Autodesk Inventor part; units mm, degrees
ref_plane "YZ Plane" through (0, 0, 0) normal (1, 0, 0) x (0, 1, 0)
ref_plane "XZ Plane" through (0, 0, 0) normal (0, 1, 0) x (-1, 0, 0)
ref_plane "XY Plane" through (0, 0, 0) normal (0, 0, 1) x (1, 0, 0)
sketch "Sketch1" plane through (0, 0, 0) normal (0, 0, 1) x (1, 0, 0)
  line L0 (-16, 16) -> (16, 16)
  line L1 (16, 16) -> (16, -16)
  line L2 (16, -16) -> (-16, -16)
  line L3 (-16, -16) -> (-16, 16)
  point P0 (0, 0)
  dimension "d0" = 32
  dimension "d1" = 32
  dimension "d2" = 16
  dimension "d3" = 16
extrude "Firkant" add sketch "Sketch1" along normal blind 6
sketch "Sketch2" plane through (0, 0, 6) normal (0, 0, 1) x (1, 0, 0)
  circle A0 centre (0, 0) radius 10.5
  dimension "d6" = 21
extrude "Rør" add sketch "Sketch2" along normal blind 51
sketch "Sketch3" plane through (0, 0, 0) normal (0, 0, -1) x (-1, 0, 0)
  circle A0 centre (0, 0) radius 6
  dimension "d9" = 12
extrude "Hul" cut sketch "Sketch3" against normal up to surface (57 mm away)
sketch "Sketch4" plane through (0, 0, 6) normal (0, 0, 1) x (1, 0, 0)
  circle A0 centre (0, 0) radius 10.5 construction
  circle A1 centre (0, 0) radius 16 construction
  line L0 (-16, 16) -> (16, -16) construction
  line L1 (16, 16) -> (-16, -16) construction
  circle A2 centre (11.3137, 11.3137) radius 2.25
  circle A3 centre (-11.3137, 11.3137) radius 2.25
  circle A4 centre (-11.3137, -11.3137) radius 2.25
  circle A5 centre (11.3137, -11.3137) radius 2.25
  dimension "d12" = 32
  dimension "d13" = 4.5
  dimension "d14" = 4.5
  dimension "d15" = 4.5
  dimension "d16" = 4.5
extrude "d1 Hullerne (små)" cut sketch "Sketch4" against normal up to surface (6 mm away)
sketch "Sketch5" plane through (0, 0, 0) normal (0, 0, -1) x (-1, 0, 0)
  circle A0 centre (11.3137, -11.3137) radius 2.25
  circle A1 centre (-11.3137, -11.3137) radius 2.25
  circle A2 centre (11.3137, 11.3137) radius 2.25
  circle A3 centre (-11.3137, 11.3137) radius 2.25
  circle A4 centre (-11.3137, 11.3137) radius 4
  circle A5 centre (11.3137, 11.3137) radius 4
  circle A6 centre (11.3137, -11.3137) radius 4
  circle A7 centre (-11.3137, -11.3137) radius 4
  dimension "d19" = 8
  dimension "d20" = 8
  dimension "d21" = 8
  dimension "d22" = 8
extrude "d2 Hullerne (store)" cut sketch "Sketch5" against normal blind 4.4
chamfer "Hjørnerne" distance 3 angle 45 4 edges at (-16, -16, 3) (16, -16, 3) (16, 16, 3) (-16, 16, 3)
equation "\"d1\" = d0"
equation "\"d14\" = d13"
equation "\"d15\" = d13"
equation "\"d16\" = d13"
equation "\"d20\" = d19"
equation "\"d21\" = d19"
equation "\"d22\" = d19"
properties part number "Z-flange" material "Aluminum 6061"
Geometry check sheet. Reference: the model listing, model coordinates, mm. A direction names the side the tool comes from. Round coordinates to 2 decimals unless told otherwise and drop trailing zeros. Loops run counter-clockwise (first coordinate to the right, second up) from the corner with the lowest first, then second, coordinate; pieces in that order, holes last. Notation, with made-up numbers: (61.5, -15) - (114.5, -15) arc R19 cw to (114.5, 4) - close; hole circle Ø7 at (-33.75, 58). An arc over 180 degrees is marked (long way). Write item = value, one per line. Start each with the question number.
1. Thickness scan on line 1 (Y direction, x = 0, z = 20); line 2 (Y direction, x = -3, z = 35.5); line 3 (X direction, y = -10, z = 4). Record the ranges inside material, lowest first.
2. Set-up check for faces 1 (the face through (-13.159, 7.765, 2.169)), 2 (the face through (10, -3.2, 31.1)), 3 (the face through (15, 14, 3)): record each of +Z, -Z, +X, -X, +Y, -Y from which the full face is reachable in a straight line by a thin tool's end or side.
3. Section check C-C on z = 43. Enter the section's corners in (x, y).
4. Mould release check, pull along Y, two halves, no side actions. Record for faces 4 (the face through (-9.168, -10.638, 5.211)), 5 (the face through (0, 16, 3)), 6 (the face through (-11, 0, 6)): released by +Y, released by -Y, zero draft, split by the parting line, or undercut.
5. Section check A-A on y = 0. Enter the section's corners in (x, z), then the cut area to 3 significant figures.
6. Depth check by flat-ended pin: pin 1 (2.5 mm diameter, centred on x = -13, y = 10.5, fed in from -Z); pin 2 (6 mm diameter, centred on y = 3.5, z = 9.5, fed in from +X); pin 3 (6 mm diameter, centred on y = 10, z = 16.5, fed in from -X); pin 4 (2.5 mm diameter, centred on x = 11.31, y = -11.31, fed in from -Z). Enter the tip coordinate at first touch or a pass-through.
Working result:
q1.line_1 = -10.5 to -6, 6 to 10.5
q1.line_2 = -10.06 to -5.2, 5.2 to 10.06
q1.line_3 = -16 to -15.09, -7.54 to 7.54, 15.09 to 16
q2.face_1 = -Z
q2.face_2 = +Z
q2.face_3 = +Z, -Z, +X, +Y
q3.outline = circle Ø21 at (0, 0); hole circle Ø12 at (0, 0)
q4.face_4 = undercut
q4.face_5 = released by +Y
q4.face_6 = zero draft
q5.outline = (-16, 0) - (-6, 0) - (-6, 57) - (-10.5, 57) - (-10.5, 6) - (-16, 6) - close; (6, 0) - (16, 0) - (16, 6) - (10.5, 6) - (10.5, 57) - (6, 57) - close
q5.area = 579 mm^2
q6.pin_1 = 4.4
q6.pin_2 = 10.49
q6.pin_3 = -7.83
q6.pin_4 = through
